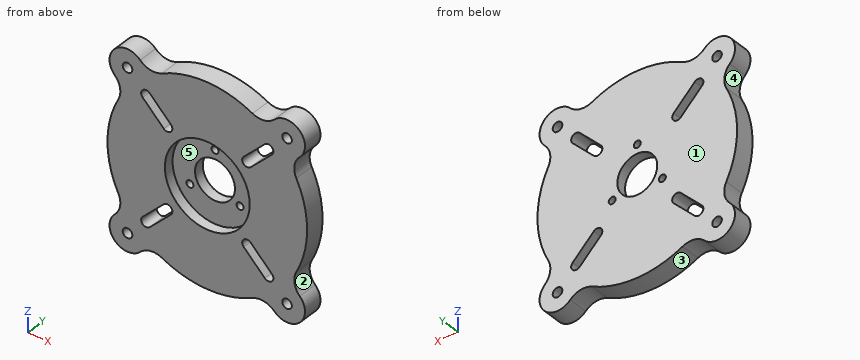
from build123d import *

# Parameters (mm, degrees)
SKETCH1_R           = 50
SKETCH1_R_2         = 2.4
BOSS_EXTRUDE2_DEPTH = 10
SKETCH2_R           = 21.25
SKETCH2_R_2         = 1.75
SKETCH2_R_3         = 10
CUT_EXTRUDE3_DEPTH  = 5
SKETCH2_2_R         = 10
SKETCH2_2_R_2       = 1.75
CUT_EXTRUDE4_DEPTH  = 11


with BuildPart() as part:
    # Sketch1 → Boss-Extrude2 (new body)
    with BuildSketch(Plane(origin=(0, 0, 0), x_dir=(1, 0, 0), z_dir=(0, 1, 0))):
        Circle(SKETCH1_R)
        with BuildLine():
            ThreePointArc((-28.838834765, 32.374368671), (-32.374368671, 32.374368671), (-32.374368671, 28.838834765))
            Line((-32.374368671, 28.838834765), (-21.767766953, 18.232233047))
            ThreePointArc((-21.767766953, 18.232233047), (-18.232233047, 18.232233047), (-18.232233047, 21.767766953))
            Line((-18.232233047, 21.767766953), (-28.838834765, 32.374368671))
        make_face(mode=Mode.SUBTRACT)
        with BuildLine():
            ThreePointArc((-32.374368671, -28.838834765), (-32.374368671, -32.374368671), (-28.838834765, -32.374368671))
            Line((-28.838834765, -32.374368671), (-18.232233047, -21.767766953))
            ThreePointArc((-18.232233047, -21.767766953), (-18.232233047, -18.232233047), (-21.767766953, -18.232233047))
            Line((-21.767766953, -18.232233047), (-32.374368671, -28.838834765))
        make_face(mode=Mode.SUBTRACT)
        with BuildLine():
            ThreePointArc((28.838834765, -32.374368671), (32.374368671, -32.374368671), (32.374368671, -28.838834765))
            Line((32.374368671, -28.838834765), (21.767766953, -18.232233047))
            ThreePointArc((21.767766953, -18.232233047), (18.232233047, -18.232233047), (18.232233047, -21.767766953))
            Line((18.232233047, -21.767766953), (28.838834765, -32.374368671))
        make_face(mode=Mode.SUBTRACT)
        with BuildLine():
            ThreePointArc((32.374368671, 28.838834765), (32.374368671, 32.374368671), (28.838834765, 32.374368671))
            Line((28.838834765, 32.374368671), (18.232233047, 21.767766953))
            ThreePointArc((18.232233047, 21.767766953), (18.232233047, 18.232233047), (21.767766953, 18.232233047))
            Line((21.767766953, 18.232233047), (32.374368671, 28.838834765))
        make_face(mode=Mode.SUBTRACT)
        with BuildLine():
            ThreePointArc((-44.576420667, 22.648238795), (-35.355339059, 35.355339059), (-22.648238795, 44.576420667))
            ThreePointArc((-22.648238795, 44.576420667), (-28.400158503, 43.670494672), (-33.587572106, 46.315494168))
            ThreePointArc((-33.587572106, 46.315494168), (-46.315494168, 46.315494168), (-46.315494168, 33.587572106))
            ThreePointArc((-46.315494168, 33.587572106), (-43.670494672, 28.400158503), (-44.576420667, 22.648238795))
        make_face()
        with Locations((-39.951533137, 39.951533137)):
            Circle(SKETCH1_R_2, mode=Mode.SUBTRACT)
        with BuildLine():
            ThreePointArc((-33.587572106, -46.315494168), (-28.400158503, -43.670494672), (-22.648238795, -44.576420667))
            ThreePointArc((-22.648238795, -44.576420667), (-35.355339059, -35.355339059), (-44.576420667, -22.648238795))
            ThreePointArc((-44.576420667, -22.648238795), (-43.670494672, -28.400158503), (-46.315494168, -33.587572106))
            ThreePointArc((-46.315494168, -33.587572106), (-46.315494168, -46.315494168), (-33.587572106, -46.315494168))
        make_face()
        with Locations((-39.951533137, -39.951533137)):
            Circle(SKETCH1_R_2, mode=Mode.SUBTRACT)
        with BuildLine():
            ThreePointArc((46.315494168, -33.587572106), (43.670494672, -28.400158503), (44.576420667, -22.648238795))
            ThreePointArc((44.576420667, -22.648238795), (35.355339059, -35.355339059), (22.648238795, -44.576420667))
            ThreePointArc((22.648238795, -44.576420667), (28.400158503, -43.670494672), (33.587572106, -46.315494168))
            ThreePointArc((33.587572106, -46.315494168), (46.315494168, -46.315494168), (46.315494168, -33.587572106))
        make_face()
        with Locations((39.951533137, -39.951533137)):
            Circle(SKETCH1_R_2, mode=Mode.SUBTRACT)
        with BuildLine():
            ThreePointArc((22.648238795, 44.576420667), (35.355339059, 35.355339059), (44.576420667, 22.648238795))
            ThreePointArc((44.576420667, 22.648238795), (43.670494672, 28.400158503), (46.315494168, 33.587572106))
            ThreePointArc((46.315494168, 33.587572106), (46.315494168, 46.315494168), (33.587572106, 46.315494168))
            ThreePointArc((33.587572106, 46.315494168), (28.400158503, 43.670494672), (22.648238795, 44.576420667))
        make_face()
        with Locations((39.951533137, 39.951533137)):
            Circle(SKETCH1_R_2, mode=Mode.SUBTRACT)
    extrude(amount=BOSS_EXTRUDE2_DEPTH)

    # Sketch2 → Cut-Extrude3 (cut)
    with BuildSketch(Plane.XZ):
        Circle(SKETCH2_R)
        with Locations((0, 14.5)):
            Circle(SKETCH2_R_2, mode=Mode.SUBTRACT)
        with Locations((12.557368355, -7.25)):
            Circle(SKETCH2_R_2, mode=Mode.SUBTRACT)
        with Locations((-12.557368355, -7.25)):
            Circle(SKETCH2_R_2, mode=Mode.SUBTRACT)
        Circle(SKETCH2_R_3, mode=Mode.SUBTRACT)
    extrude(amount=-CUT_EXTRUDE3_DEPTH, mode=Mode.SUBTRACT)

    # Sketch2_2 → Cut-Extrude4 (cut, through all)
    with BuildSketch(Plane.XZ):
        Circle(SKETCH2_2_R)
        with Locations((-12.557368355, -7.25)):
            Circle(SKETCH2_2_R_2)
        with Locations((0, 14.5)):
            Circle(SKETCH2_2_R_2)
        with Locations((12.557368355, -7.25)):
            Circle(SKETCH2_2_R_2)
    extrude(amount=-CUT_EXTRUDE4_DEPTH, mode=Mode.SUBTRACT)


solid = part.part
The model under review builds one solid part; all positions refer to its coordinate system, in mm. Face numbers are marked on the shaded views. A direction names the side the tool comes from. Round coordinates to 2 decimals unless told otherwise and drop trailing zeros. Loops run counter-clockwise (first coordinate to the right, second up) from the corner with the lowest first, then second, coordinate; pieces in that order, holes last. Notation, with made-up numbers: M 37,29.25 L 50,29.25 A9 ccw 50,45.25 Z; hole C 46.25,-22 d1. An arc over 180 degrees is marked long. Answer as a JSON object with one key per item and string values.
Item 1: We need section B-B, the plane z = -24. State the section outline as (x, y) points.
Check sheet entries:
{"outline": "M -44.02,0 L -27.54,0 L -27.54,10 L -44.02,10 Z; M -20.46,0 L 20.46,0 L 20.46,10 L -20.46,10 Z; M 27.54,0 L 44.02,0 L 44.02,10 L 27.54,10 Z"}
Item 2: We need section D-D, the plane y = 2. State how many separate pieces and enclosed holes the cut face has, and give its area (3 significant figures).
Check sheet entries:
{"separate pieces": "1", "enclosed holes": "9", "area": "7,060 mm2"}
Item 3: The part is to be moulded in two halves that separate along X. For the marked faces 1, 2 and 3, say which applies: +X half, -X half, draft (parallel to the pull), parting line (faces both ways), or undercut.
Check sheet entries:
{"face 1": "draft", "face 2": "+X half", "face 3": "undercut"}
Item 4: Tool access review of the marked faces 4 and 5: name each direction out of +Z, -Z, +X, -X, +Y, -Y from which nothing blocks a thin tool from reaching the whole face with its end or side.
Check sheet entries:
{"face 4": "-X, +Y, -Y", "face 5": "-Y"}
Item 5: Clearance check with flat-ended pins moving along their axes: P1, Ø5, axis at y = 1.5, z = -37, coming from the -X side; P2, Ø1, axis at x = -8.5, y = 7.5, coming from the +Z side; P3, Ø4, axis at x = 12.56, z = -7.25, coming from the -Y side. State where each tip first meets the part, or that it passes through.
Check sheet entries:
{"P1": "x = -48.94", "P2": "z = 49.36", "P3": "y = 5"}
Item 6: We need section A-A, the plane x = 0. State the section outline as (y, z) points, and give its area (3 significant figures).
Check sheet entries:
{"outline": "M 0,-50 L 10,-50 L 10,-10 L 5,-10 L 5,-21.25 L 0,-21.25 Z; M 0,21.25 L 5,21.25 L 5,16.25 L 10,16.25 L 10,50 L 0,50 Z; M 5,10 L 10,10 L 10,12.75 L 5,12.75 Z", "area": "670 mm2"}
Item 7: We need section C-C, the plane z = 6.5. State the section outline as (x, y) points, and give its area (3 significant figures).
Check sheet entries:
{"outline": "M -49.58,0 L -20.23,0 L -20.23,5 L -7.6,5 L -7.6,10 L -49.58,10 Z; M 7.6,5 L 20.23,5 L 20.23,0 L 49.58,0 L 49.58,10 L 7.6,10 Z", "area": "713 mm2"}
Item 8: For line 1 along Z through (x, y) = (29.5, 9.5); line 2 along Z through (x, y) = (29, 1.75); line 3 along X through (y, z) = (6.5, -21), list the stretches that pass through material, from the lowest coordinate up.
Check sheet entries:
{"line 1": "-43.91 to -32.85, -25.96 to 25.96, 32.85 to 43.91", "line 2": "-43.79 to -32.52, -25.46 to 25.46, 32.52 to 43.79", "line 3": "-45.38 to -24.54, -17.71 to 17.71, 24.54 to 45.38"}
